Source: CAD feature listing. Evaluate the final solid. Frame: model axes, mm. Give positions to 0.01 mm unless a question says otherwise; leave off trailing zeros. Write each loop counter-clockwise with the first axis right and the second up, starting at its lowest first coordinate (ties: lowest second). Pieces come first, ordered by that corner, then holes. Notation, with made-up numbers: M 5,86.25 L 16,86.25 A30 ccw 16,108.25 Z; hole C 81,67.5 d4. An arc over 180 degrees is marked long. Return JSON: item names as keys, results as strings.
```python
from build123d import *

# Parameters (mm, degrees)
F0_W     = 19.05
F0_H     = 152.4
F0_W_2   = 152.4
F0_H_2   = 19.05
F1_DEPTH = 19.05


with BuildPart() as f1:
    # F0 (on Front) → F1 (new body)
    with BuildSketch(Plane.XZ):
        with Locations((-693.232657, -177.8)):
            Rectangle(F0_W, F0_H)
        with Locations((767.267343, -177.8)):
            Rectangle(F0_W, F0_H)
        with Locations((-328.107657, -365.125)):
            Rectangle(F0_W_2, F0_H_2)
        with Locations((402.142343, -365.125)):
            Rectangle(F0_W_2, F0_H_2)
        Polygon((-683.707657, -254), (-683.707657, -355.6), (-404.307657, -355.6), (-251.907657, -355.6), (325.942343, -355.6), (478.342343, -355.6), (757.742343, -355.6), (757.742343, -254), (757.742343, -101.6), (757.742343, 0), (776.792343, 0), (776.792343, 514.35), (548.192343, 514.35), (395.792343, 514.35), (-321.757657, 514.35), (-474.157657, 514.35), (-702.757657, 514.35), (-702.757657, 0), (-683.707657, 0), (-683.707657, -101.6), align=None)
        with Locations((37.017343, -171.45)):
            Rectangle(F0_W, F0_H, mode=Mode.SUBTRACT)
        with Locations((-328.107657, -9.525)):
            Rectangle(F0_W_2, F0_H_2, mode=Mode.SUBTRACT)
        with Locations((402.142343, -9.525)):
            Rectangle(F0_W_2, F0_H_2, mode=Mode.SUBTRACT)
        with Locations((-397.957657, 523.875)):
            Rectangle(F0_W_2, F0_H_2)
        with Locations((471.992343, 523.875)):
            Rectangle(F0_W_2, F0_H_2)
    extrude(amount=F1_DEPTH)


solid = f1.part
```
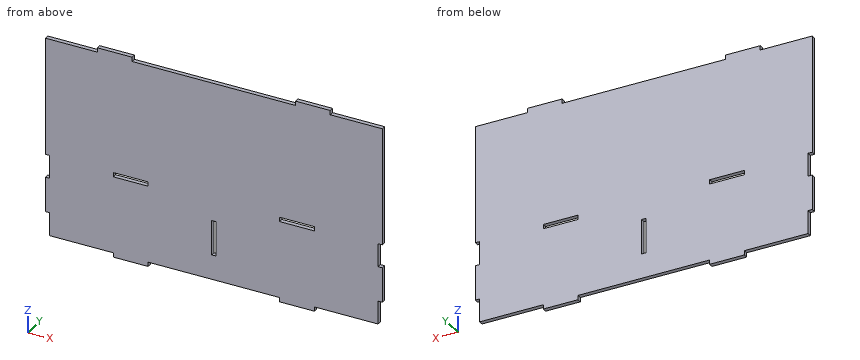
1) Cut plane C-C, the plane z = -317. Return the cut outline in (x, y).
Numbers:
{"outline": "M -683.71,-19.05 L 757.74,-19.05 L 757.74,0 L -683.71,0 Z"}
2) Cut plane B-B, the plane x = -140. Return the cut outline in (y, z), then the cut area to 3 significant figures.
Numbers:
{"outline": "M -19.05,-355.6 L 0,-355.6 L 0,514.35 L -19.05,514.35 Z", "area": "16,600 mm²"}
3) Line query: line 1 (X direction, y = -13.75, z = -3); line 2 (X direction, y = -9, z = -244.5); line 3 (Z direction, x = 448.5, y = -5.25). Output: solid intervals per line, ascending. Write a range as [from, to].
Numbers:
{"line 1": "x = [-683.71, -404.31], [-251.91, 325.94], [478.34, 757.74]", "line 2": "x = [-702.76, 27.49], [46.54, 776.79]", "line 3": "z = [-374.65, -19.05], [0, 533.4]"}
4) Cut plane A-A, the plane y = -8.25. Give the number of separate pieces and of enclosed holes in the cut face, then the cut area to 3 significant figures.
Numbers:
{"separate pieces": "1", "enclosed holes": "3", "area": "1,280,000 mm²"}
5) Contact query for flat-ended pins moving along their axis: pin 1 Ø6 at (y, z) = (-13.5, -267.5) entering from +X; pin 2 Ø5.5 at (x, y) = (364.5, -13.5) entering from +Z; pin 3 Ø5.5 at (y, z) = (-9, -324) entering from -X. Output: stop coordinate, or through.
Numbers:
{"pin 1": "stops at x = 757.74", "pin 2": "stops at z = 514.35", "pin 3": "stops at x = -683.71"}
